The listing builds one solid part. Answer for the finished solid, in the listing's coordinates (mm). Face numbers are marked on the shaded views. A direction names the side the tool comes from. Coordinates: 2 decimals unless noted, no trailing zeros. One line per item, written item: value. Start each with the question number.
Q1. Straight lines are drawn through the part: line 1 along Z through (x, y) = (-0.25, 0) (3 decimals); line 2 along Z through (x, y) = (0.5, 10); line 3 along Z through (x, y) = (7, -11). For each, find the intervals that lie inside material, in ascending order. Write a range as [from, to].
Q2. Determine the mould class of the marked faces 3, 4, 5 and 6 for opening direction Z: pulls with the +Z half, pulls with the -Z half, needs draft (parallel to the pull), parting line crosses it, or undercut.
Q3. The part is cut by section A-A on y = 0. Give the number of separate pieces and of enclosed holes in the cut face, then the cut area to 3 significant figures.
Q4. For the marked faces 1 and 2, determine the directions among +Z, -Z, +X, -X, +Y, -Y from which every point of the face is accessible in a straight line to the end or side of a thin tool.
Q5. Each of these flat-tipped pins is pushed along its axis until it touches: pin 1 Ø10 at (y, z) = (-21, -25) entering from -X; pin 2 Ø4 at (x, z) = (8, -12.5) entering from -Y; pin 3 Ø5 at (y, z) = (-10, 23) entering from +X; pin 4 Ø1.5 at (y, z) = (21, -1) entering from +X. Where does it stop, or does it pass through?
```python
from build123d import *

# Parameters (mm, degrees)
F0_R             = 26.924
F1_DEPTH         = 5.08
F2_R             = 31.75
F3_DEPTH         = 10.16
F4_R             = 8.001
F5_DEPTH         = 15.241
F6_SIZE          = 0.762
F7_R             = 5.08
F8_DEPTH         = 15.241
F8_COPIES_COUNT  = 8
F9_R             = 3.175
F10_DEPTH        = 7.62
F10_COPIES_COUNT = 8
F11_SIZE         = 0.762


# Not quite as in the source:
# - a pattern or mirror of a feature is missing from the dataset's text; its kind, count and spacing are read off the source's solid


with BuildPart() as f1:
    # F0 (on Right) → F1 (new body)
    with BuildSketch(Plane.YZ):
        Circle(F0_R)
    extrude(amount=-F1_DEPTH)

    # F2 (on face) → F3 (join)
    with BuildSketch(Plane.YZ):
        Circle(F2_R)
    extrude(amount=F3_DEPTH)

    # F4 (on face) → F5 (cut, through all)
    with BuildSketch(Plane.YZ.offset(10.16)):
        Circle(F4_R)
    extrude(amount=-F5_DEPTH, mode=Mode.SUBTRACT)

    # F6
    f6_edges = [f1.edges().sort_by_distance(p)[0] for p in [
        (10.16, -8.001, 0),
        (10.16, -31.75, 0),
        (0, -31.75, 0),
        (-5.08, -26.924, 0),
        (-5.08, -8.001, 0),
    ]]
    chamfer(f6_edges, length=F6_SIZE)

    # F7 (on face) → F8 (cut, through all)
    with BuildSketch(Plane(origin=(-5.08, 0, 0), x_dir=(0, -1, 0), z_dir=(-1, 0, 0))):
        with Locations((0, 18.415)):
            Circle(F7_R)
    f8 = extrude(amount=-F8_DEPTH, mode=Mode.SUBTRACT)

    # F8_copies: F8 ×8 about axis
    f8_copies_axis = Axis((0, 0, 0), (1, 0, 0))
    for i in range(1, F8_COPIES_COUNT):
        add(f8.rotate(f8_copies_axis, i * 360 / F8_COPIES_COUNT), mode=Mode.SUBTRACT)

    # F9 (on face) → F10 (cut)
    with BuildSketch(Plane.YZ.offset(10.16)):
        with Locations((-9.7201591821, 23.4665401258)):
            Circle(F9_R)
    f10 = extrude(amount=-F10_DEPTH, mode=Mode.SUBTRACT)

    # F10_copies: F10 ×8 about axis
    f10_copies_axis = Axis((0, 0, 0), (1, 0, 0))
    for i in range(1, F10_COPIES_COUNT):
        add(f10.rotate(f10_copies_axis, i * 360 / F10_COPIES_COUNT), mode=Mode.SUBTRACT)

    # F11
    f11_edges = [f1.edges().sort_by_distance(p)[0] for p in [
        (10.16, -12.895159, 23.46654),
        (10.16, 5.08, 18.415),
        (-5.08, 5.08, 18.415),
        (10.16, -7.475095, -25.711604),
        (10.16, -23.46654, -12.895159),
        (10.16, -16.613474, -9.429269),
        (10.16, 12.895159, -23.46654),
        (10.16, -5.08, -18.415),
        (10.16, 9.429269, -16.613474),
        (10.16, 25.711604, -7.475095),
        (10.16, 18.415, -5.08),
        (10.16, -18.415, 5.08),
        (10.16, -25.711604, 7.475095),
        (10.16, -9.429269, 16.613474),
        (10.16, 16.613474, 9.429269),
        (10.16, 23.46654, 12.895159),
        (10.16, 7.475095, 25.711604),
        (-5.08, -16.613474, -9.429269),
        (-5.08, -5.08, -18.415),
        (-5.08, 9.429269, -16.613474),
        (-5.08, 18.415, -5.08),
        (-5.08, -18.415, 5.08),
        (-5.08, -9.429269, 16.613474),
        (-5.08, 16.613474, 9.429269),
    ]]
    chamfer(f11_edges, length=F11_SIZE)


solid = f1.part
```
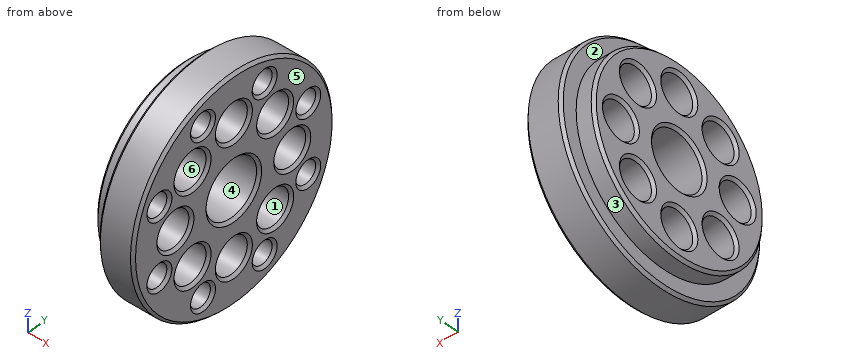
Output:
1. line 1: z = [-26.924, -23.495], [-13.335, -8.001], [8.001, 13.335], [23.495, 26.924]
1. line 2: z = [-29.86, -17.11], [-8.94, 8.94], [17.11, 29.86]
1. line 3: z = [-29.78, -26.37], [-20.56, -17.68], [-8.36, 8.36], [17.68, 20.56], [26.37, 29.78]
2. face 3: parting line crosses it
2. face 4: undercut
2. face 5: needs draft
2. face 6: undercut
3. separate pieces: 4
3. enclosed holes: 0
3. area: 360 mm^2
4. face 1: +X, -X
4. face 2: -X
5. pin 1: stops at x = 0
5. pin 2: stops at y = -29.96
5. pin 3: stops at x = 2.54
5. pin 4: passes through
